```python
from build123d import *

# Parameters (mm, degrees)
ESQUISSE1_W                  = 30
ESQUISSE1_H                  = 30
BOSS_EXTRU_1_DEPTH           = 12
ENL_V_MAT_EXTRU_1_DEPTH      = 45.09081537
ENL_V_MAT_EXTRU_1_DEPTH_BACK = 45.09081537
ESQUISSE2_R                  = 2
ENL_V_MAT_EXTRU_2_DEPTH      = 45.09081537
ENL_V_MAT_EXTRU_2_DEPTH_BACK = 45.09081537
ESQUISSE3_W                  = 20
ESQUISSE3_H                  = 20
CONG_1_R                     = 5


with BuildPart() as part:
    # Esquisse1 → Boss.-Extru.1 (new body)
    with BuildSketch(Plane.XY):
        with Locations((15, 15)):
            Rectangle(ESQUISSE1_W, ESQUISSE1_H)
    extrude(amount=BOSS_EXTRU_1_DEPTH)

    # Esquisse2 → Enlèv. mat.-Extru.1 (cut, two sides: drawn at the far end of the back side and taken through both)
    with BuildSketch(Plane.XY.offset(12).offset(-ENL_V_MAT_EXTRU_1_DEPTH_BACK)):
        with Locations((5, 25)):
            Circle(ESQUISSE2_R)
        with Locations(Location((25, 25, 0), (0, 0, 180))):
            Circle(ESQUISSE2_R)
        with Locations((25, 5)):
            Circle(ESQUISSE2_R)
        with Locations(Location((5, 5, 0), (0, 0, 180))):
            Circle(ESQUISSE2_R)
    extrude(amount=ENL_V_MAT_EXTRU_1_DEPTH + ENL_V_MAT_EXTRU_1_DEPTH_BACK, mode=Mode.SUBTRACT)

    # Esquisse3 → Enlèv. mat.-Extru.2 (cut, two sides: drawn at the far end of the back side and taken through both)
    with BuildSketch(Plane.XY.offset(12).offset(-ENL_V_MAT_EXTRU_2_DEPTH_BACK)):
        with Locations((20, 10)):
            Rectangle(ESQUISSE3_W, ESQUISSE3_H)
    extrude(amount=ENL_V_MAT_EXTRU_2_DEPTH + ENL_V_MAT_EXTRU_2_DEPTH_BACK, mode=Mode.SUBTRACT)

    # Congé1
    cong_1_edges = [part.edges().sort_by_distance(p)[0] for p in [
        (10, 20, 6),
        (0, 30, 6),
        (0, 0, 6),
        (10, 0, 6),
        (30, 30, 6),
        (30, 20, 6),
    ]]
    fillet(cong_1_edges, radius=CONG_1_R - 0.0001)  # a hair under: the kernel refuses the full size


solid = part.part
```
Design review of the part built by this model. Coordinates are the model's own, in mm. A direction names the side the tool comes from. Coordinates: 2 decimals unless noted, no trailing zeros. Order: outer loops, then holes, each group sorted by start corner. A loop starts at its lowest first (then second) coordinate and runs counter-clockwise, first axis right, second up.
1) Take a section at D-D, the plane y = 9. Give the boundary of the cut face in (x, z).
2) Take a section at C-C, the plane x = 8. Give the boundary of the cut face in (y, z).
3) Take a section at A-A, the plane z = 5.5. State how many separate pieces and enclosed holes the cut face has, and give its area (3 significant figures).
4) Clearance check with flat-ended pins moving along their axes: pin 1 (1.5 mm diameter, centred on y = 12, z = 4, fed in from +X); pin 2 (3 mm diameter, centred on x = 20, z = 3.5, fed in from -Y). State where each tip first meets the part, or that it passes through.
5) Wall thickness on line 1 along Y through (x, z) = (5, 9.5); line 2 along Y through (x, z) = (25, 4); line 3 along Y through (x, z) = (18.25, 3): over which ranges is each line inside the solid? List them lowest first.
6) Take a section at B-B, the plane y = 3.75. Give the boundary of the cut face in (x, z), and give its area (3 significant figures).
7) Mouldability with a two-part tool opening along X and no side actions: class faces 3 (the flat face through (20, 20, 6)), 4 (the cylindrical face through (29, 22, 6)), 5 (the cylindrical face through (6.6, 6.2, 5.9)) as +X half, -X half, draft (parallel to the pull), parting line (faces both ways), or undercut.
8) For faces 1 (the cylindrical face through (26.6, 26.2, 5.9)), 2 (the flat face through (10, 10, 6)), list the 3-axis set-ups (+Z, -Z, +X, -X, +Y, -Y) from which the entire face can be reached by the end or side of a thin tool; tool diameter is ignored.
Returned:
1. outline: (0, 0) - (10, 0) - (10, 12) - (0, 12) - close
2. outline: (1, 0) - (30, 0) - (30, 12) - (1, 12) - close
3. separate pieces: 1
3. enclosed holes: 3
3. area: 441 mm2
4. pin 1: stops at x = 10
4. pin 2: stops at y = 20
5. line 1: y = 0 to 3, 7 to 23, 27 to 30
5. line 2: y = 20 to 23, 27 to 30
5. line 3: y = 20 to 30
6. outline: (0.16, 0) - (3.44, 0) - (3.44, 12) - (0.16, 12) - close; (6.56, 0) - (9.84, 0) - (9.84, 12) - (6.56, 12) - close
6. area: 78.7 mm2
7. face 3: draft
7. face 4: +X half
7. face 5: undercut
8. face 1: +Z, -Z
8. face 2: +Z, -Z, +X, -Y
